For this review, take the finished solid that the model builds, in its own axes (mm). A direction names the side the tool comes from. Give positions to 0.01 mm unless a question says otherwise; leave off trailing zeros. Order: outer loops, then holes, each group sorted by start corner. A loop starts at its lowest first (then second) coordinate and runs counter-clockwise, first axis right, second up. Notation, with made-up numbers: (8, 32) - (66, 32) arc R33 cw to (66, 67) - close; hole circle Ø3 at (-14, 81). An arc over 180 degrees is marked (long way). Use a Markdown table: item, result. Add a question column.
1) We need section C-C on z = 0. Write out the cut boundary in (x, y).
2) We need section B-B on x = 7.5. Write out the cut boundary in (y, z), then the cut area to 3 significant figures.
3) Clearance check with flat-ended pins moving along their axes: P1, Ø12, axis at y = 22, z = 4, coming from the +X side; P2, Ø3, axis at x = -2, z = 9.5, coming from the +Y side; P3, Ø3, axis at y = 28.5, z = -13, coming from the -X side; P4, Ø7, axis at x = 7.5, y = 32, coming from the -Z side. State where each tip first meets the part, or that it passes through.
4) Machinability: for faces 1 (the face through (4, 30, -12.5)), 2 (the face through (7, 58, -17)), which of the approach directions +Z, -Z, +X, -X, +Y, -Y give a long, thin tool a straight path to every point of the face, cutting with its end or side? Answer none if there is none.
5) We need section A-A on y = 41. Write out the cut boundary in (x, z), then the cut area to 3 significant figures.
6) Wall thickness on L1, parallel to Z at x = 10, y = 12.5; L2, parallel to Y at x = 7.5, z = 14; L3, parallel to X at y = 42.5, z = -3: over which ranges is each line inside the solid? List them lowest first.
7) We need section D-D on y = 34. Write out the cut boundary in (x, z).
8) Mouldability with a two-part tool opening along X and no side actions: class faces 3 (the face through (7, 27, -20)), 4 (the face through (10.27, 30.85, -16.2)), 5 (the face through (-15.239, 59.757, 0.335)), 6 (the face through (10.27, 30.85, 16.3)) as released by +X, released by -X, zero draft, split by the parting line, or undercut.
```python
from build123d import *

# Parameters (mm, degrees)
SALIENTE_EXTRUIR1_DEPTH = 60
CHAFL_N1_SIZE           = 5
CROQUIS2_R              = 3
CORTAR_EXTRUIR1_DEPTH   = 40


with BuildPart() as part:
    # Croquis1 → Saliente-Extruir1 (new body)
    with BuildSketch(Plane(origin=(0, 0, 0), x_dir=(1, 0, 0), z_dir=(0, 1, 0))):
        with BuildLine():
            Line((0, 20), (15, 20))
            ThreePointArc((15, 20), (35, 0), (15, -20))
            Line((15, -20), (0, -20))
            ThreePointArc((0, -20), (-20, 0), (0, 20))
        make_face()
        with BuildLine():
            Line((0, 12.5), (15, 12.5))
            ThreePointArc((15, 12.5), (27.5, 0), (15, -12.5))
            Line((15, -12.5), (0, -12.5))
            ThreePointArc((0, -12.5), (-12.5, 0), (0, 12.5))
        make_face(mode=Mode.SUBTRACT)
    extrude(amount=SALIENTE_EXTRUIR1_DEPTH)

    # Chaflán1
    chafl_n1_edges = [part.edges().sort_by_distance(p)[0] for p in [
        (35, 60, 0),
        (7.5, 60, -20),
        (-20, 60, 0),
        (7.5, 60, 20),
    ]]
    chamfer(chafl_n1_edges, length=CHAFL_N1_SIZE)

    # Croquis2 → Cortar-Extruir1 (cut)
    with BuildSketch(Plane.XY.offset(20)):
        with Locations((7.5, 32)):
            Circle(CROQUIS2_R)
    extrude(amount=-CORTAR_EXTRUIR1_DEPTH, mode=Mode.SUBTRACT)


solid = part.part
```
Checked values:
| question | item | result |
|---|---|---|
| 1 | outline | (-20, 0) - (-12.5, 0) - (-12.5, 60) - (-15, 60) - (-20, 55) - close; (27.5, 0) - (35, 0) - (35, 55) - (30, 60) - (27.5, 60) - close |
| 2 | outline | (0, -20) - (29, -20) - (29, -12.5) - (0, -12.5) - close; (0, 12.5) - (29, 12.5) - (29, 20) - (0, 20) - close; (35, -20) - (55, -20) - (60, -15) - (60, -12.5) - (35, -12.5) - close; (35, 12.5) - (60, 12.5) - (60, 15) - (55, 20) - (35, 20) - close |
| 2 | area | 785 mm² |
| 3 | P1 | x = 35 |
| 3 | P2 | through |
| 3 | P3 | x = -16.36 |
| 3 | P4 | z = -20 |
| 4 | face 1 | +Y, -Y |
| 4 | face 2 | -Z, +X, -X, +Y |
| 5 | outline | (0, -20) - (15, -20) arc R20 ccw to (15, 20) - (0, 20) arc R20 ccw to start; hole (0, -12.5) - (15, -12.5) arc R12.5 ccw to (15, 12.5) - (0, 12.5) arc R12.5 ccw to start |
| 5 | area | 991 mm² |
| 6 | L1 | -20 to -12.5, 12.5 to 20 |
| 6 | L2 | 0 to 29, 35 to 60 |
| 6 | L3 | -19.77 to -12.13, 27.13 to 34.77 |
| 7 | outline | (0, -20) - (5.26, -20) - (5.26, -12.5) - (0, -12.5) arc R12.5 cw to (0, 12.5) - (5.26, 12.5) - (5.26, 20) - (0, 20) arc R20 ccw to start; (9.74, -20) - (15, -20) arc R20 ccw to (15, 20) - (9.74, 20) - (9.74, 12.5) - (15, 12.5) arc R12.5 cw to (15, -12.5) - (9.74, -12.5) - close |
| 8 | face 3 | zero draft |
| 8 | face 4 | undercut |
| 8 | face 5 | released by -X |
| 8 | face 6 | undercut |
